Job drawing, mm, ordinate dimensions from the low corner. One solid piece. A direction names the side the tool comes from. Round coordinates to 2 decimals unless told otherwise and drop trailing zeros. Loops run counter-clockwise (first coordinate to the right, second up) from the corner with the lowest first, then second, coordinate; pieces in that order, holes last.
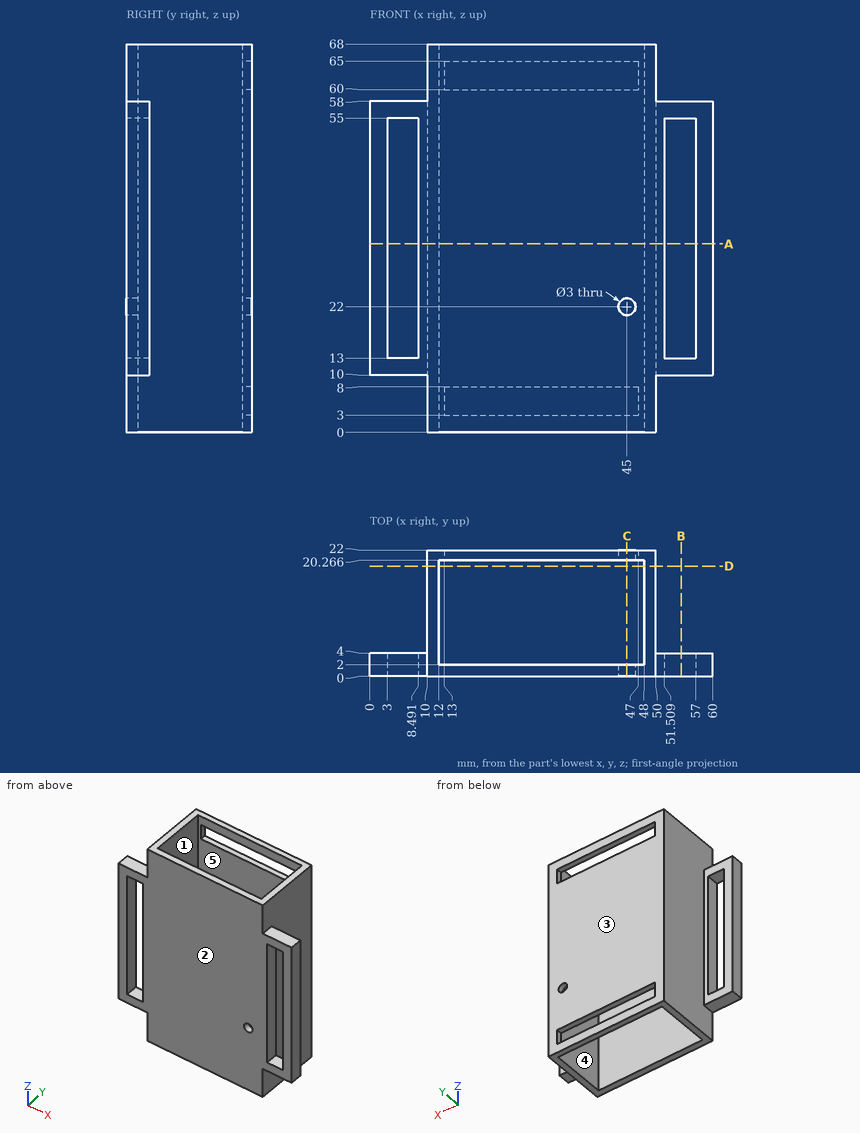
(1) Probe line 1 (Z direction, x = 45, y = 20.95); line 2 (X direction, y = 1.5, z = 16); line 3 (X direction, y = 0.4, z = 22). List the from-to ranges inside material, lowest first.
Responses:
line 1: z = 0 to 3, 8 to 20.5, 23.5 to 60, 65 to 68
line 2: x = 0 to 3, 8.49 to 51.51, 57 to 60
line 3: x = 0 to 3, 8.49 to 43.5, 46.5 to 51.51, 57 to 60
(2) Which spindle directions (+Z, -Z, +X, -X, +Y, -Y) get a long thin tool onto all of the face, cutting with end or side? Do the marked faces 1 and 2. Say none if no direction does.
Responses:
face 1: +Z, -Z
face 2: +Z, -Z, +X, -X, -Y
(3) Pull direction X, two halves, no side cores. Call the marked faces 3, 4 and 5: +X half, -X half, draft (parallel to the pull), parting line (faces both ways), or undercut.
Responses:
face 3: draft
face 4: undercut
face 5: undercut
(4) Slice it at C-C on x = 45. List the corners of the cut face in (y, z), plus the area to 3 significant figures.
Responses:
outline: (0, 0) - (2, 0) - (2, 20.5) - (0, 20.5) - close; (0, 23.5) - (2, 23.5) - (2, 68) - (0, 68) - close; (20.27, 0) - (22, 0) - (22, 3) - (20.27, 3) - close; (20.27, 8) - (22, 8) - (22, 20.5) - (20.27, 20.5) - close; (20.27, 23.5) - (22, 23.5) - (22, 60) - (20.27, 60) - close; (20.27, 65) - (22, 65) - (22, 68) - (20.27, 68) - close
area: 225 mm2
(5) Slice it at A-A on z = 33. List the corners of the cut face in (x, y).
Responses:
outline: (0, 0) - (3, 0) - (3, 4) - (0, 4) - close; (8.49, 0) - (51.51, 0) - (51.51, 4) - (50, 4) - (50, 22) - (10, 22) - (10, 4) - (8.49, 4) - close; (57, 0) - (60, 0) - (60, 4) - (57, 4) - close; hole (12, 2) - (48, 2) - (48, 20.27) - (12, 20.27) - close
(6) Slice it at D-D on y = 19.25. List the corners of the cut face in (x, z), plus the area to 3 significant figures.
Responses:
outline: (10, 0) - (12, 0) - (12, 68) - (10, 68) - close; (48, 0) - (50, 0) - (50, 68) - (48, 68) - close
area: 272 mm2
(7) Slice it at B-B on x = 54.5. List the corners of the cut face in (y, z), plus the area to 3 significant figures.
Responses:
outline: (0, 10) - (4, 10) - (4, 13) - (0, 13) - close; (0, 55) - (4, 55) - (4, 58) - (0, 58) - close
area: 24.0 mm2
(8) Pin check, flat tips, straight feed: P1, Ø1.2, axis at x = 6.5, y = 1.5, coming from the -Z side; P2, Ø4.5, axis at x = 6, y = 2.5, coming from the +Z side; P3, Ø6.5, axis at y = 12.5, z = 40, coming from the +X side. Stop position of each tip, or through.
Responses:
P1: stops at z = 10
P2: stops at z = 58
P3: stops at x = 50
